Answer from the drawing. Dimensions are ordinates in mm from the lowest x, y and z of the part. A direction names the side the tool comes from. Coordinates: 2 decimals unless noted, no trailing zeros. Write each loop counter-clockwise with the first axis right and the second up, starting at its lowest first coordinate (ties: lowest second). Pieces come first, ordered by that corner, then holes.
(1) Which of the six approach directions +Z, -Z, +X, -X, +Y, -Y give full straight-line access (tool end or side, diameter ignored) to the marked faces 5 and 6?
(2) The part is cut by section C-C, the plane y = 30.5. Determine the outline of the cut face in (x, z), and give its area (3 significant figures).
(3) Straight lines are drawn through the part: line 1 along Z through (x, y) = (38, 13.5); line 2 along X through (y, z) = (18, 29); line 3 along X through (y, z) = (8, 52.5). For each, find the intervals that lie inside material, in ascending order.
(4) Given pin 1 (8 mm diameter, centred on x = 39, y = 3.5, fed in from -Z), flat-ended and moving along its own axis, determine where the tip first touches the part or whether it passes through.
(5) The part is cut by section A-A, the plane x = 32. Determine the outline of the cut face in (y, z).
(6) Determine the mould class of the marked faces 1, 2, 3 and 4 for opening direction X: pulls with the +X half, pulls with the -X half, needs draft (parallel to the pull), parting line crosses it, or undercut.
(7) The part is cut by section B-B, the plane z = 24. Determine the outline of the cut face in (x, y), and give its area (3 significant figures).
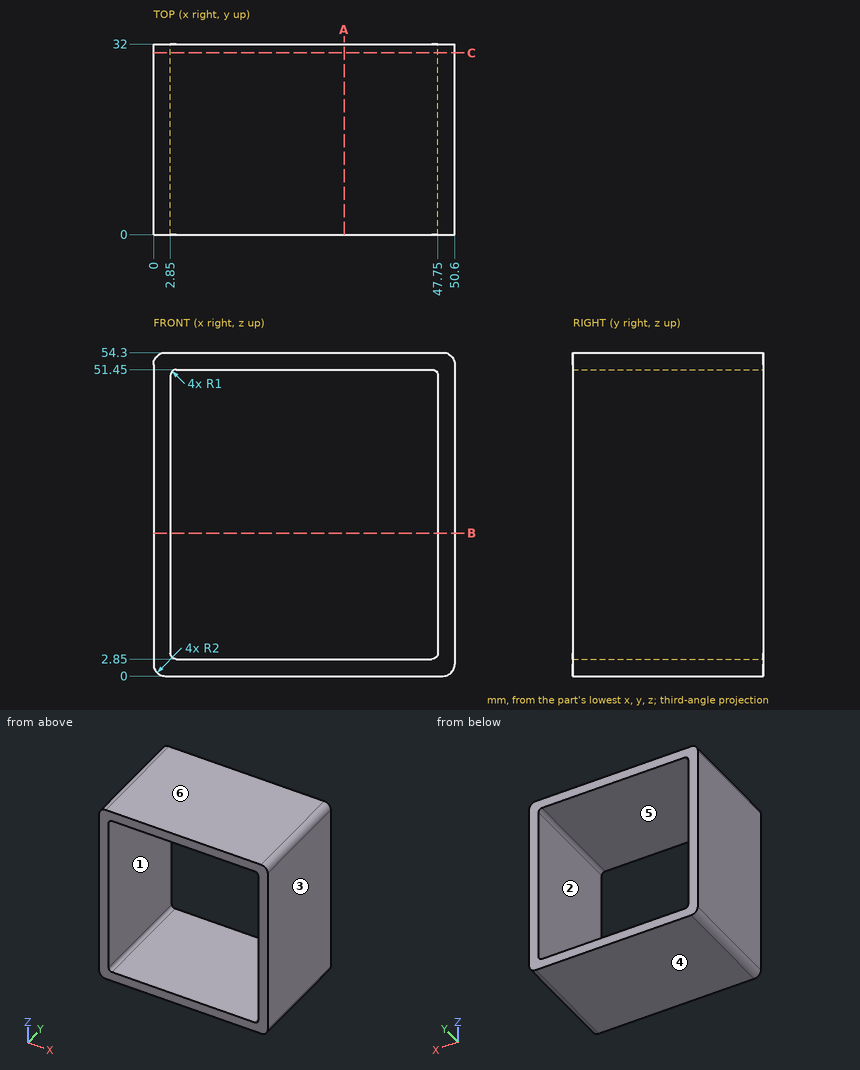
Computed:
1. face 5: +Y, -Y
1. face 6: +Z, +X, -X, +Y, -Y
2. outline: (0, 2) arc R2 ccw to (2, 0) - (48.6, 0) arc R2 ccw to (50.6, 2) - (50.6, 52.3) arc R2 ccw to (48.6, 54.3) - (2, 54.3) arc R2 ccw to (0, 52.3) - close; hole (2.85, 3.85) arc R1 ccw to (3.85, 2.85) - (46.75, 2.85) arc R1 ccw to (47.75, 3.85) - (47.75, 50.45) arc R1 ccw to (46.75, 51.45) - (3.85, 51.45) arc R1 ccw to (2.85, 50.45) - close
2. area: 563 mm2
3. line 1: z = 0 to 2.85, 51.45 to 54.3
3. line 2: x = 0 to 2.85, 47.75 to 50.6
3. line 3: x = 0.01 to 50.59
4. pin 1: stops at z = 0
5. outline: (0, 0) - (32, 0) - (32, 2.85) - (0, 2.85) - close; (0, 51.45) - (32, 51.45) - (32, 54.3) - (0, 54.3) - close
6. face 1: undercut
6. face 2: undercut
6. face 3: pulls with the +X half
6. face 4: needs draft
7. outline: (0, 0) - (2.85, 0) - (2.85, 32) - (0, 32) - close; (47.75, 0) - (50.6, 0) - (50.6, 32) - (47.75, 32) - close
7. area: 182 mm2
